Drawing for the job (mm, zero at the part's lowest x, y, z). Give positions to 0.01 mm unless a question says otherwise; leave off trailing zeros. Write each loop counter-clockwise with the first axis right and the second up, starting at its lowest first coordinate (ties: lowest second). Pieces come first, ordered by that corner, then holes.
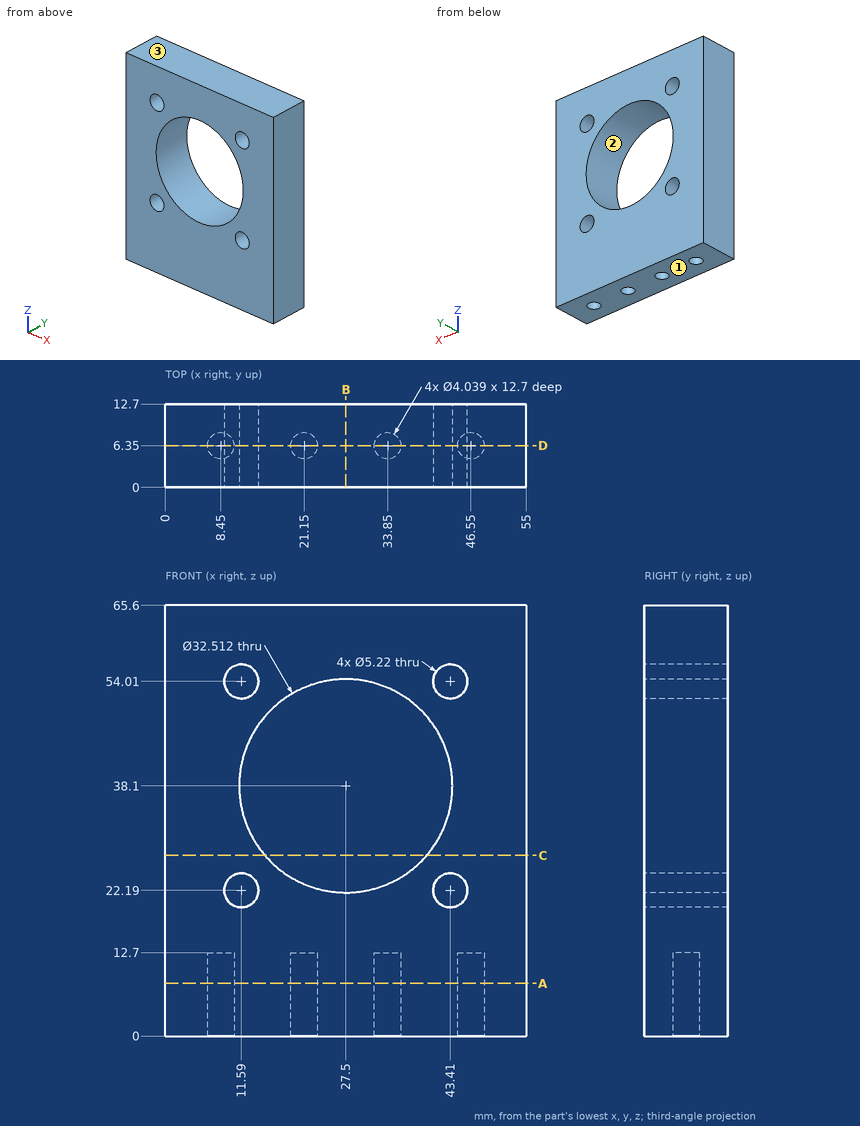
1. Slice it at B-B, the plane x = 27.5. Write the cut outline in (y, z), and give its area (3 significant figures).
Calculated:
outline: (0, 0) - (12.7, 0) - (12.7, 21.84) - (0, 21.84) - close; (0, 54.36) - (12.7, 54.36) - (12.7, 65.6) - (0, 65.6) - close
area: 420 mm2
2. Pin check, flat tips, straight feed: P1, Ø2, axis at x = 46, y = 7, coming from the -Z side; P2, Ø3, axis at x = 43.41, z = 22.19, coming from the -Y side. Stop position of each tip, or through.
Calculated:
P1: stops at z = 12.7
P2: passes through
3. Probe probe 1 along X at (y, z) = (9.5, 55.5); probe 2 along X at (y, z) = (3.75, 55) (1 decimal); probe 3 along Z at (x, y) = (45.5, 1) (1 decimal). List the from-to ranges inside material, lowest first.
Calculated:
probe 1: x = 0 to 9.45, 13.73 to 41.27, 45.55 to 55
probe 2: x = 0 to 9.2, 14 to 41, 45.8 to 55
probe 3: z = 0 to 20.6, 23.8 to 52.4, 55.6 to 65.6
4. Slice it at D-D, the plane y = 6.35. Write the cut outline in (x, z), and give its area (3 significant figures).
Calculated:
outline: (0, 0) - (6.43, 0) - (6.43, 12.7) - (10.47, 12.7) - (10.47, 0) - (19.13, 0) - (19.13, 12.7) - (23.17, 12.7) - (23.17, 0) - (31.83, 0) - (31.83, 12.7) - (35.87, 12.7) - (35.87, 0) - (44.53, 0) - (44.53, 12.7) - (48.57, 12.7) - (48.57, 0) - (55, 0) - (55, 65.6) - (0, 65.6) - close; hole circle Ø5.22 at (11.59, 22.19); hole circle Ø5.22 at (11.59, 54.01); hole circle Ø32.51 at (27.5, 38.1); hole circle Ø5.22 at (43.41, 22.19); hole circle Ø5.22 at (43.41, 54.01)
area: 2,490 mm2
5. Slice it at C-C, the plane z = 27.5. Write the cut outline in (x, y) (1 decimal).
Calculated:
outline: (0, 0) - (15.2, 0) - (15.2, 12.7) - (0, 12.7) - close; (39.8, 0) - (55, 0) - (55, 12.7) - (39.8, 12.7) - close
6. Slice it at A-A, the plane z = 8. Write the cut outline in (x, y), and give its area (3 significant figures).
Calculated:
outline: (0, 0) - (55, 0) - (55, 12.7) - (0, 12.7) - close; hole circle Ø4.04 at (8.45, 6.35); hole circle Ø4.04 at (21.15, 6.35); hole circle Ø4.04 at (33.85, 6.35); hole circle Ø4.04 at (46.55, 6.35)
area: 647 mm2
7. Pull direction Z, two halves, no side cores. Call the marked faces 1, 2 and 3: +Z half, -Z half, draft (parallel to the pull), parting line (faces both ways), or undercut.
Calculated:
face 1: -Z half
face 2: undercut
face 3: +Z half
